from build123d import *

# Parameters (mm, degrees)
ESTRUSIONE_ESTRUSIONE1_DEPTH = 1.35
SCHIZZO2_R                   = 3.375
ESTRUSIONE_ESTRUSIONE2_DEPTH = 2
SCHIZZO3_R                   = 2.25
TAGLIO_ESTRUSIONE1_DEPTH     = 2
SCHIZZO4_R                   = 1
TAGLIO_ESTRUSIONE2_DEPTH     = 9.910141694


with BuildPart() as part:
    # Schizzo1 → Estrusione-Estrusione1 (new body)
    with BuildSketch(Plane(origin=(0, 0, 0), x_dir=(1, 0, 0), z_dir=(0, 1, 0))):
        with BuildLine():
            Line((8, 2.102337115), (2.090005981, 2.65))
            ThreePointArc((2.090005981, 2.65), (3.036807138, 1.472558117), (3.375, 0))
            ThreePointArc((3.375, 0), (3.036807138, -1.472558117), (2.090005981, -2.65))
            Line((2.090005981, -2.65), (8, -2.102337115))
            Line((8, -2.102337115), (8, 2.102337115))
        make_face()
        with BuildLine():
            ThreePointArc((2.090005981, 2.65), (0, 3.375), (-2.090005981, 2.65))
            Line((-2.090005981, 2.65), (-2.090005981, -2.65))
            ThreePointArc((-2.090005981, -2.65), (0, -3.375), (2.090005981, -2.65))
            Line((2.090005981, -2.65), (2.090005981, 2.65))
        make_face()
        with BuildLine():
            ThreePointArc((-2.090005981, -2.65), (-3.375, 0), (-2.090005981, 2.65))
            Line((-2.090005981, 2.65), (-8, 2.102337115))
            Line((-8, 2.102337115), (-8, -2.102337115))
            Line((-8, -2.102337115), (-2.090005981, -2.65))
        make_face()
        with BuildLine():
            Line((-2.090005981, -2.65), (-2.090005981, 2.65))
            ThreePointArc((-2.090005981, 2.65), (-3.375, 0), (-2.090005981, -2.65))
        make_face()
        with BuildLine():
            ThreePointArc((3.375, 0), (3.036807138, 1.472558117), (2.090005981, 2.65))
            Line((2.090005981, 2.65), (2.090005981, -2.65))
            ThreePointArc((2.090005981, -2.65), (3.036807138, -1.472558117), (3.375, 0))
        make_face()
    extrude(amount=ESTRUSIONE_ESTRUSIONE1_DEPTH)

    # Schizzo2 → Estrusione-Estrusione2 (add)
    with BuildSketch(Plane(origin=(0, 1.35, 0), x_dir=(1, 0, 0), z_dir=(0, 1, 0))):
        with Locations(Location((0, 0, 0), (0, 0, 51.737808872))):
            Circle(SCHIZZO2_R)
    extrude(amount=ESTRUSIONE_ESTRUSIONE2_DEPTH)

    # Schizzo3 → Taglio-Estrusione1 (cut)
    with BuildSketch(Plane(origin=(0, 3.35, 0), x_dir=(1, 0, 0), z_dir=(0, 1, 0))):
        with Locations(Location((0, 0, 0), (0, 0, 270))):
            Circle(SCHIZZO3_R)
    extrude(amount=-TAGLIO_ESTRUSIONE1_DEPTH, mode=Mode.SUBTRACT)

    # Schizzo4 → Taglio-Estrusione2 (cut, through all)
    with BuildSketch(Plane(origin=(0, 1.35, 0), x_dir=(1, 0, 0), z_dir=(0, 1, 0))):
        with Locations(Location((0, 0, 0), (0, 0, 270))):
            Circle(SCHIZZO4_R)
    extrude(amount=-TAGLIO_ESTRUSIONE2_DEPTH, mode=Mode.SUBTRACT)


solid = part.part
Can you work these out from the model? Positions are in its coordinate system, mm. Coordinates: 2 decimals unless noted, no trailing zeros. Order: outer loops, then holes, each group sorted by start corner. A loop starts at its lowest first (then second) coordinate and runs counter-clockwise, first axis right, second up. Notation, with made-up numbers: M 27,81.5 L 75,81.5 A16 cw 75,107.5 Z; hole C 87,77 d3. An arc over 180 degrees is marked long. Write item = value, one per line.
(1) Suppose I cut it at D-D on z = -0.75. Please give me the cut outline in (x, y).
Results are:
outline = M -8,0 L -0.66,0 L -0.66,1.35 L -2.12,1.35 L -2.12,3.35 L -3.29,3.35 L -3.29,1.35 L -8,1.35 Z; M 0.66,0 L 8,0 L 8,1.35 L 3.29,1.35 L 3.29,3.35 L 2.12,3.35 L 2.12,1.35 L 0.66,1.35 Z
(2) Suppose I cut it at C-C on z = 0. Please give me the cut outline in (x, y) (3 decimals), plus the area to 3 significant figures.
Results are:
outline = M -8,0 L -1,0 L -1,1.35 L -2.25,1.35 L -2.25,3.35 L -3.375,3.35 L -3.375,1.35 L -8,1.35 Z; M 1,0 L 8,0 L 8,1.35 L 3.375,1.35 L 3.375,3.35 L 2.25,3.35 L 2.25,1.35 L 1,1.35 Z
area = 23.4 mm2
(3) Suppose I cut it at B-B on y = 0.85. Please give me the cut outline in (x, z) (3 decimals), plus the area to 3 significant figures.
Results are:
outline = M -8,-2.102 L -2.09,-2.65 A3.375 ccw 2.09,-2.65 L 8,-2.102 L 8,2.102 L 2.09,2.65 A3.375 ccw -2.09,2.65 L -8,2.102 Z; hole C 0,0 d2
area = 79.3 mm2
(4) I need wall thicknesses on line 1 along X through (y, z) = (2.4, 0) (3 decimals); line 2 along X through (y, z) = (0.5, 0); line 3 along Y through (x, z) = (-7.25, 0.25). Which ranges of each line are inside material? Lowest first, please. Write a range as [from, to].
Results are:
line_1 = [-3.375, -2.25], [2.25, 3.375]
line_2 = [-8, -1], [1, 8]
line_3 = [0, 1.35]
(5) If we mould it in two halves opening along Z, with no side actions, what happens to faces 1 (the face through (-5.09, 0.67, 2.37)), 2 (the face through (0.676, 2.364, 2.146)), 3 (the face through (8, 1, 0)), 4 (the face through (-1, 1.35, -1))? For each: pulls with the +Z half, pulls with the -Z half, needs draft (parallel to the pull), parting line crosses it, or undercut.
Results are:
face_1 = pulls with the +Z half
face_2 = undercut
face_3 = needs draft
face_4 = undercut
(6) For pin 1 Ø1.5 at (y, z) = (3, -0.5) entering from -X (3 decimals); pin 2 Ø1 at (y, z) = (2, -1.5) entering from +X; pin 3 Ø2.5 at (x, z) = (-6, 0) entering from +Y, each with a flat end and sliding along its axis, tell me the tip position at first contact or that it passes through.
Results are:
pin_1 = -3.375
pin_2 = 3.22
pin_3 = 1.35
(7) Suppose I cut it at A-A on x = 0. Please give me the cut outline in (y, z) (3 decimals), plus the area to 3 significant figures.
Results are:
outline = M 0,-3.375 L 3.35,-3.375 L 3.35,-2.25 L 1.35,-2.25 L 1.35,-1 L 0,-1 Z; M 0,1 L 1.35,1 L 1.35,2.25 L 3.35,2.25 L 3.35,3.375 L 0,3.375 Z
area = 10.9 mm2
